```python
from build123d import *

# Parameters (mm, degrees)
F3_D     = 4.2
F5_DEPTH = 10


with BuildPart() as f1:
    # F0 (on Front) → F1 (revolve)
    with BuildSketch(Plane.XZ):
        Polygon((-5, 0), (0, 0), (0, 2), (-3, 2), (-3.5, 15), (-6, 15), (-5, 8), align=None)
    revolve(axis=Axis((0, 0, 1), (0, 0, 1)))

    # F3 (through all)
    with Locations(Plane(origin=(0, 0, 0), x_dir=(1, 0, 0), z_dir=(0, 0, -1))):
        with Locations((0, 0)):
            Hole(F3_D / 2)

    # F4 (on face) → F5 (cut)
    with BuildSketch(Plane.XY.offset(15)):
        with BuildLine():
            Line((-2.0396078054, 0.5), (-3.4641016151, 0.5))
            ThreePointArc((-3.4641016151, 0.5), (-3.5, 0), (-3.4641016151, -0.5))
            Line((-3.4641016151, -0.5), (-2.0396078054, -0.5))
            ThreePointArc((-2.0396078054, -0.5), (-2.1, 0), (-2.0396078054, 0.5))
        make_face()
        with BuildLine():
            Line((-3.4641016151, 0.5), (-5.9791303716, 0.5))
            ThreePointArc((-5.9791303716, 0.5), (-6, 0), (-5.9791303716, -0.5))
            Line((-5.9791303716, -0.5), (-3.4641016151, -0.5))
            ThreePointArc((-3.4641016151, -0.5), (-3.5, 0), (-3.4641016151, 0.5))
        make_face()
        with BuildLine():
            ThreePointArc((0.5, 3.4641016151), (0, 3.5), (-0.5, 3.4641016151))
            Line((-0.5, 3.4641016151), (-0.5, 2.0396078054))
            ThreePointArc((-0.5, 2.0396078054), (0, 2.1), (0.5, 2.0396078054))
            Line((0.5, 2.0396078054), (0.5, 3.4641016151))
        make_face()
        with BuildLine():
            ThreePointArc((0.5, 5.9791303716), (0, 6), (-0.5, 5.9791303716))
            Line((-0.5, 5.9791303716), (-0.5, 3.4641016151))
            ThreePointArc((-0.5, 3.4641016151), (0, 3.5), (0.5, 3.4641016151))
            Line((0.5, 3.4641016151), (0.5, 5.9791303716))
        make_face()
        with BuildLine():
            ThreePointArc((3.5, 0), (3.491013868, 0.2506435188), (3.4641016151, 0.5))
            Line((3.4641016151, 0.5), (2.0396078054, 0.5))
            ThreePointArc((2.0396078054, 0.5), (2.1, 0), (2.0396078054, -0.5))
            Line((2.0396078054, -0.5), (3.4641016151, -0.5))
            ThreePointArc((3.4641016151, -0.5), (3.491013868, -0.2506435188), (3.5, 0))
        make_face()
        with BuildLine():
            ThreePointArc((6, 0), (5.9947803225, 0.2502176759), (5.9791303716, 0.5))
            Line((5.9791303716, 0.5), (3.4641016151, 0.5))
            ThreePointArc((3.4641016151, 0.5), (3.491013868, 0.2506435188), (3.5, 0))
            ThreePointArc((3.5, 0), (3.491013868, -0.2506435188), (3.4641016151, -0.5))
            Line((3.4641016151, -0.5), (5.9791303716, -0.5))
            ThreePointArc((5.9791303716, -0.5), (5.9947803225, -0.2502176759), (6, 0))
        make_face()
        with BuildLine():
            Line((-0.5, -2.0396078054), (-0.5, -3.4641016151))
            ThreePointArc((-0.5, -3.4641016151), (0, -3.5), (0.5, -3.4641016151))
            Line((0.5, -3.4641016151), (0.5, -2.0396078054))
            ThreePointArc((0.5, -2.0396078054), (0, -2.1), (-0.5, -2.0396078054))
        make_face()
        with BuildLine():
            Line((-0.5, -3.4641016151), (-0.5, -5.9791303716))
            ThreePointArc((-0.5, -5.9791303716), (0, -6), (0.5, -5.9791303716))
            Line((0.5, -5.9791303716), (0.5, -3.4641016151))
            ThreePointArc((0.5, -3.4641016151), (0, -3.5), (-0.5, -3.4641016151))
        make_face()
    extrude(amount=-F5_DEPTH, mode=Mode.SUBTRACT)


solid = f1.part
```
Input: part model. Units: mm. Frame: model coordinates. A direction names the side the tool comes from. Round coordinates to 2 decimals unless told otherwise and drop trailing zeros. Loops run counter-clockwise (first coordinate to the right, second up) from the corner with the lowest first, then second, coordinate; pieces in that order, holes last. Notation, with made-up numbers: (-29.75, 17) -> (-11.75, 17) arc R23 ccw to (-11.75, 40) -> close; hole circle Ø7 at (81, 52.5). An arc over 180 degrees is marked (long way). Use one line per item in the form item = value. Start each with the question number.
Item 1: Mould query, pull axis X, two halves, no side actions, for faces 1 (the face through (-3.85, 3.92, 11.45)), 2 (the face through (-4.619, 1.915, 3.944)), 3 (the face through (4, -0.5, 10)), 4 (the face through (1.3, 2, 2)). Classes: pulls with the +X half, pulls with the -X half, needs draft (parallel to the pull), parting line crosses it, or undercut.
Item 2: Section query D-D on z = 5.25. Return the cut outline in (x, y) (3 decimals), then the cut area to 3 significant figures.
Item 3: Section query A-A on z = 10.75. Return the cut outline in (x, y).
Item 4: Section query B-B on x = 0. Return the cut outline in (y, z).
Item 5: Set-up query: faces 5 (the face through (-1.501, 2.886, 8.591)), 6 (the face through (-4, 0, 5)), 7 (the face through (0.5, -4, 10)). Return all of +Z, -Z, +X, -X, +Y, -Y with unobstructed straight access to the full face (end or side cutting, diameter ignored); none if empty.
Item 6: Contact query for flat-ended pins moving along their axis: pin 1 Ø0.9 at (x, z) = (4, 9) entering from -Y; pin 2 Ø6 at (x, z) = (-1.5, 3) entering from +Y; pin 3 Ø2.5 at (x, z) = (-4.5, 10) entering from -Y. Output: stop coordinate, or through.
Item 7: Material intervals for L1, parallel to Y at x = 0, z = 0.4; L2, parallel to Z at x = -1.75, y = -2; L3, parallel to X at y = -2, z = 8, sorted ascending. Write a range as from..to.
Ans:
q1.face_1 = pulls with the -X half
q1.face_2 = parting line crosses it
q1.face_3 = needs draft
q1.face_4 = undercut
q2.outline = (-4.975, -0.5) arc R5 ccw to (-0.5, -4.975) -> (-0.5, -3.085) arc R3.125 cw to (-3.085, -0.5) -> close; (-4.975, 0.5) -> (-3.085, 0.5) arc R3.125 cw to (-0.5, 3.085) -> (-0.5, 4.975) arc R5 ccw to start; (0.5, -4.975) arc R5 ccw to (4.975, -0.5) -> (3.085, -0.5) arc R3.125 cw to (0.5, -3.085) -> close; (0.5, 3.085) arc R3.125 cw to (3.085, 0.5) -> (4.975, 0.5) arc R5 ccw to (0.5, 4.975) -> close
q2.area = 40.3 mm^2
q3.outline = (-5.37, -0.5) arc R5.39 ccw to (-0.5, -5.37) -> (-0.5, -3.3) arc R3.34 cw to (-3.3, -0.5) -> close; (-5.37, 0.5) -> (-3.3, 0.5) arc R3.34 cw to (-0.5, 3.3) -> (-0.5, 5.37) arc R5.39 ccw to start; (0.5, -5.37) arc R5.39 ccw to (5.37, -0.5) -> (3.3, -0.5) arc R3.34 cw to (0.5, -3.3) -> close; (0.5, 3.3) arc R3.34 cw to (3.3, 0.5) -> (5.37, 0.5) arc R5.39 ccw to (0.5, 5.37) -> close
q4.outline = (-5, 0) -> (-2.1, 0) -> (-2.1, 2) -> (-3, 2) -> (-3.12, 5) -> (-5, 5) -> close; (2.1, 0) -> (5, 0) -> (5, 5) -> (3.12, 5) -> (3, 2) -> (2.1, 2) -> close
q5.face_5 = +Z
q5.face_6 = +Z, +X, -X
q5.face_7 = +Z, +Y, -Y
q6.pin_1 = -3.73
q6.pin_2 = 5
q6.pin_3 = -4.19
q7.L1 = -5..-2.1, 2.1..5
q7.L2 = 0..2
q7.L3 = -4.58..-2.54, 2.54..4.58
